Geometry: final body of the model. Coordinates: model frame, mm. A direction names the side the tool comes from. Give positions to 0.01 mm unless a question says otherwise; leave off trailing zeros. Write each loop counter-clockwise with the first axis right and the second up, starting at its lowest first coordinate (ties: lowest second). Pieces come first, ordered by that corner, then holes. Notation, with made-up numbers: M 1.5,-18.75 L 58.5,-18.75 A23 ccw 58.5,-8.75 Z; hole C -29,81.25 d4. An arc over 180 degrees is marked long. One line per question, with ' | ' between items.
from build123d import *

# Parameters (mm, degrees)
F0_W     = 5.842
F0_H     = 12.7
F1_DEPTH = 20.574
F2_R     = 5.08
F3_R     = 5.07999
F0_R     = 3.175
F4_DEPTH = 10.668
F5_R     = 1.5253482573
F6_DEPTH = 4.826


# Not quite as in the source:
# - a fillet or chamfer is up to 0.001 mm smaller than in the source, because OpenCascade refuses the exact size


with BuildPart() as f1:
    # F0 (on Front) → F1 (new body)
    with BuildSketch(Plane.XZ):
        Polygon((5.842, 12.7), (5.842, 0), (66.294, 0), (66.294, 12.7), (56.134, 12.7), (56.134, 10.16), (10.16, 10.16), (10.16, 12.7), align=None)
        with Locations((2.921, 6.35)):
            Rectangle(F0_W, F0_H)
    extrude(amount=F1_DEPTH)

    # F2
    f2_edges = [f1.edges().sort_by_distance(p)[0] for p in [
        (33.147, 0, 10.16),
        (33.147, -20.574, 10.16),
    ]]
    fillet(f2_edges, radius=F2_R)

    # F3 (radius 5.08 in the source; OpenCascade refuses exactly that, so slightly less here)
    f3_edges = [f1.edges().sort_by_distance(p)[0] for p in [
        (33.147, 0, 0),
        (61.214, 0, 12.7),
        (61.214, -20.574, 12.7),
        (5.08, 0, 12.7),
        (5.08, -20.574, 12.7),
        (33.147, -20.574, 0),
    ]]
    fillet(f3_edges, radius=F3_R)

    # F0 (on Front) → F4 (join)
    with BuildSketch(Plane.XZ):
        with BuildLine():
            ThreePointArc((-8.1826630726, -5.5069827884), (-3.1957909266, -4.5493385486), (-0.9398, 0))
            ThreePointArc((-0.9398, 0), (-4.5919612295, 5.3297205562), (-10.8806298187, 3.8475430269))
            ThreePointArc((-10.8806298187, 3.8475430269), (-12.1459778134, -1.5837270034), (-8.1826630726, -5.5069827884))
        make_face()
        with Locations((-6.6548, 0)):
            Circle(F0_R, mode=Mode.SUBTRACT)
        with BuildLine():
            Line((-0.9398, 0), (0, 0))
            Line((0, 0), (0, 12.7))
            Line((0, 12.7), (5.842, 12.7))
            Line((5.842, 12.7), (5.842, 15.24))
            Line((5.842, 15.24), (-0.508, 15.24))
            Line((-0.508, 15.24), (-10.8806298187, 3.8475430269))
            ThreePointArc((-10.8806298187, 3.8475430269), (-4.5919612295, 5.3297205562), (-0.9398, 0))
        make_face()
    extrude(amount=F4_DEPTH)

    # F5 (on face) → F6 (join)
    with BuildSketch(Plane.YZ.offset(66.294)):
        with BuildLine():
            Line((-15.49401, 12.7), (-5.6335453628, 12.7))
            Line((-5.6335453628, 12.7), (-5.6335453628, 15.2267941305))
            Line((-5.6335453628, 15.2267941305), (-14.7798256949, 15.2267941305))
            Line((-14.7798256949, 15.2267941305), (-15.7828871161, 15.2267941305))
            Line((-15.7828871161, 15.2267941305), (-15.7713881355, 12.6924216326))
            ThreePointArc((-15.7713881355, 12.6924216326), (-15.632750821, 12.6981050547), (-15.49401, 12.7))
        make_face()
        with BuildLine():
            ThreePointArc((-15.7424642816, 6.3176113686), (-10.7967240539, 11.3957731119), (-5.6335453628, 6.5388544493))
            Line((-5.6335453628, 6.5388544493), (-5.6335453628, 12.7))
            Line((-5.6335453628, 12.7), (-15.49401, 12.7))
            ThreePointArc((-15.49401, 12.7), (-15.632750821, 12.6981050547), (-15.7713881355, 12.6924216326))
            Line((-15.7713881355, 12.6924216326), (-15.7424642816, 6.3176113686))
        make_face()
        with BuildLine():
            ThreePointArc((-15.7424642816, 6.3176113686), (-10.6746149155, 1.2841357749), (-5.6296554142, 6.3405532201))
            ThreePointArc((-5.6296554142, 6.3405532201), (-5.6306279949, 6.4397229095), (-5.6335453628, 6.5388544493))
            ThreePointArc((-5.6335453628, 6.5388544493), (-10.7967240539, 11.3957731119), (-15.7424642816, 6.3176113686))
        make_face()
        with Locations((-10.6860858708, 6.3405532201)):
            Circle(F5_R, mode=Mode.SUBTRACT)
    extrude(amount=F6_DEPTH)


solid = f1.part
(1) Material intervals for L1, parallel to X at y = -17.75, z = 12; L2, parallel to Z at x = 22, y = -12.25; L3, parallel to X at y = -10, z = 10.75, sorted ascending. Write a range as [from, to].
Working result:
L1: x = [0, 10.16], [56.13, 66.29] | L2: z = [0, 10.16] | L3: x = [-4.6, 10.16], [56.13, 71.12]
(2) Cut plane A-A, the plane y = -8. Return loops of the section in (x, z) (3 decimals), then the cut area to 3 significant figures.
Working result:
outline: M -10.881,3.848 A5.715 ccw long -0.94,0 L 66.294,0 L 66.294,2.057 L 71.12,2.057 L 71.12,15.227 L 66.294,15.227 L 66.294,12.7 L 56.134,12.7 L 56.134,10.16 L 10.16,10.16 L 10.16,12.7 L 5.842,12.7 L 5.842,15.24 L -0.508,15.24 Z; hole C -6.655,0 d6.35 | area: 934 mm^2
(3) First-contact query: P1, Ø2.5, axis at y = -2, z = 9.5, coming from the +X side; P2, Ø8, axis at y = -15, z = 5, coming from the -X side; P3, Ø4, axis at x = 1.5, y = -3, coming from the -Z side. Flat tips, straight axial feed; report the tip coordinate or a pass-through.
Working result:
P1: stops at x = 66.29 | P2: stops at x = 0 | P3: stops at z = 0
(4) Cut plane B-B, the plane z = 9. Return loops of the section in (x, y), then the cut area to 3 significant figures.
Working result:
outline: M -6.19,-10.67 L 0,-10.67 L 0,-20.38 L 10.16,-20.38 L 10.16,-18.73 L 56.13,-18.73 L 56.13,-20.38 L 66.29,-20.38 L 66.29,-15.75 L 71.12,-15.75 L 71.12,-5.63 L 66.29,-5.63 L 66.29,-0.19 L 56.13,-0.19 L 56.13,-1.85 L 10.16,-1.85 L 10.16,-0.19 L 0,-0.19 L 0,0 L -6.19,0 Z | area: 1,300 mm^2
(5) Cut plane C-C, the plane y = -3.5. Return loops of the section in (x, z) (3 decimals), then the cut area to 3 significant figures.
Working result:
outline: M -10.881,3.848 A5.715 ccw long -0.94,0 L 0,0 L 0,0.252 L 66.294,0.252 L 66.294,12.448 L 56.134,12.448 L 56.134,9.908 L 10.16,9.908 L 10.16,12.448 L 0,12.448 L 0,12.7 L 5.842,12.7 L 5.842,15.24 L -0.508,15.24 Z; hole C -6.655,0 d6.35 | area: 837 mm^2
(6) Set-up query: faces 1 (the face through (66.294, -5.6, 4.8)), 2 (the face through (0, -1, 11)), 3 (the face through (32.825, -1.528, 8.711)), 4 (the face through (5.842, -5, 14)), 5 (the face through (61.143, -1.528, 11.251)). Return all of +Z, -Z, +X, -X, +Y, -Y with unobstructed straight access to the full face (end or side cutting, diameter ignored); none if empty.
Working result:
face 1: -Z, +X | face 2: +X, +Y | face 3: +Z, +Y | face 4: +Z, +Y, -Y | face 5: +Z, +X, +Y
